from build123d import *

# Parameters (mm, degrees)
SKETCH1_W           = 35
SKETCH1_H           = 12
BOSS_EXTRUDE1_DEPTH = 25
SKETCH2_R           = 5
CUT_EXTRUDE1_DEPTH  = 18
SKETCH3_R           = 2.1
CUT_EXTRUDE2_DEPTH  = 15
SKETCH4_R           = 1.5
CUT_EXTRUDE3_DEPTH  = 7
SKETCH5_R           = 1.75
CUT_EXTRUDE4_DEPTH  = 13
SKETCH6_R           = 4
CUT_EXTRUDE5_DEPTH  = 4


with BuildPart() as part:
    # Sketch1 → Boss-Extrude1 (new body)
    with BuildSketch(Plane(origin=(0, 0, 0), x_dir=(1, 0, 0), z_dir=(0, 1, 0))):
        Rectangle(SKETCH1_W, SKETCH1_H)
    extrude(amount=BOSS_EXTRUDE1_DEPTH)

    # Sketch2 → Cut-Extrude1 (cut)
    with BuildSketch(Plane.XZ):
        Circle(SKETCH2_R)
    extrude(amount=-CUT_EXTRUDE1_DEPTH, mode=Mode.SUBTRACT)

    # Sketch3 → Cut-Extrude2 (cut)
    with BuildSketch(Plane(origin=(0, 25, 0), x_dir=(1, 0, 0), z_dir=(0, 1, 0))):
        with Locations((-5, 0)):
            Circle(SKETCH3_R)
        with Locations((5, 0)):
            Circle(SKETCH3_R)
    extrude(amount=-CUT_EXTRUDE2_DEPTH, mode=Mode.SUBTRACT)

    # Sketch4 → Cut-Extrude3 (cut)
    with BuildSketch(Plane.XY.offset(6)):
        with Locations((0, 12)):
            Circle(SKETCH4_R)
    extrude(amount=-CUT_EXTRUDE3_DEPTH, mode=Mode.SUBTRACT)

    # Sketch5 → Cut-Extrude4 (cut, through all)
    with BuildSketch(Plane.XY.offset(6)):
        with Locations((-12.5, 15)):
            Circle(SKETCH5_R)
        with Locations((12.5, 15)):
            Circle(SKETCH5_R)
    extrude(amount=-CUT_EXTRUDE4_DEPTH, mode=Mode.SUBTRACT)

    # Sketch6 → Cut-Extrude5 (cut)
    with BuildSketch(Plane.XY.offset(6)):
        with Locations((-12.5, 15)):
            Circle(SKETCH6_R)
        with Locations((12.5, 15)):
            Circle(SKETCH6_R)
    extrude(amount=-CUT_EXTRUDE5_DEPTH, mode=Mode.SUBTRACT)


solid = part.part
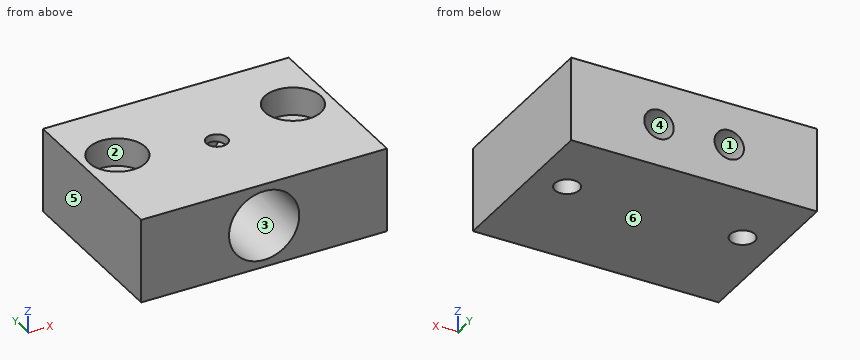
Input: part model. Units: mm. Frame: model coordinates. Face numbers are marked on the shaded views. A direction names the side the tool comes from. Give positions to 0.01 mm unless a question says otherwise; leave off trailing zeros. Loops run counter-clockwise (first coordinate to the right, second up) from the corner with the lowest first, then second, coordinate; pieces in that order, holes last. Notation, with made-up numbers: M -7.5,82.5 L 20.5,82.5 A16 cw 20.5,92.5 Z; hole C 34.5,1.25 d3. An arc over 180 degrees is marked long. Use one line per item in the form item = value.
1. Line query: L1, parallel to X at y = 9, z = 0; L2, parallel to X at y = 23, z = 0; L3, parallel to X at y = 15.75, z = 0. Output: solid intervals per line, ascending.
Numbers:
L1 = -17.5 to -5, 5 to 17.5
L2 = -17.5 to -7.1, -2.9 to 2.9, 7.1 to 17.5
L3 = -17.5 to -14.08, -10.92 to -7.1, 7.1 to 10.92, 14.08 to 17.5
2. Reachability of the marked faces 1, 2 and 3 from +Z, -Z, +X, -X, +Y, -Y: full face, straight path, thin tool, end or side. Return the list, or none.
Numbers:
face_1 = +Y
face_2 = +Z
face_3 = -Y
3. Section query C-C, the plane z = 4. Return the cut outline in (x, y).
Numbers:
outline = M -17.5,0 L -3,0 L -3,18 L 3,18 L 3,0 L 17.5,0 L 17.5,25 L -17.5,25 Z; hole C -12.5,15 d8; hole C 12.5,15 d8
4. Section query A-A, the plane z = 0. Return the cut outline in (x, y).
Numbers:
outline = M -17.5,0 L -5,0 L -5,10 L -7.1,10 L -7.1,25 L -17.5,25 Z; M -2.9,18 L 2.9,18 L 2.9,25 L -2.9,25 Z; M 5,0 L 17.5,0 L 17.5,25 L 7.1,25 L 7.1,10 L 5,10 Z; hole C -12.5,15 d3.5; hole C 12.5,15 d3.5
5. First-contact query: pin 1 (6 mm diameter, centred on x = 14, z = -4, fed in from -Y); pin 2 (4 mm diameter, centred on x = -13.5, y = 16.5, fed in from +Z); pin 3 (1.3 mm diameter, centred on x = -5.5, z = -1, fed in from +Y); pin 4 (2.5 mm diameter, centred on x = 1, z = 1, fed in from -Y). Flat tips, straight axial feed; report the tip coordinate or a pass-through.
Numbers:
pin_1 = 0
pin_2 = 2
pin_3 = 10
pin_4 = 18
6. Section query B-B, the plane x = 0. Return the cut outline in (y, z).
Numbers:
outline = M 0,-6 L 25,-6 L 25,6 L 13.5,6 L 13.5,5 L 18,5 L 18,-5 L 0,-5 Z; M 0,5 L 10.5,5 L 10.5,6 L 0,6 Z
7. Pull-direction query (Z, two-part tool) for the marked faces 4, 5 and 6; classes: released by +Z, released by -Z, zero draft, split by the parting line, or undercut.
Numbers:
face_4 = undercut
face_5 = zero draft
face_6 = released by -Z
8. Section query D-D, the plane y = 19.5. Return the cut outline in (x, z).
Numbers:
outline = M -17.5,-6 L 17.5,-6 L 17.5,6 L -17.5,6 Z; hole C -5,0 d4.2; hole C 5,0 d4.2
